Check sheet for the drawn part. Datum: minimum x, y, z corner. Units: mm. A direction names the side the tool comes from. Round coordinates to 2 decimals unless told otherwise and drop trailing zeros. Order: outer loops, then holes, each group sorted by start corner. A loop starts at its lowest first (then second) coordinate and runs counter-clockwise, first axis right, second up. Notation, with made-up numbers: (72, 50) -> (93, 50) arc R21 cw to (93, 65) -> close; hole circle Ø11 at (33.25, 89). An arc over 180 degrees is marked (long way). Answer in a Markdown table with one row per item.
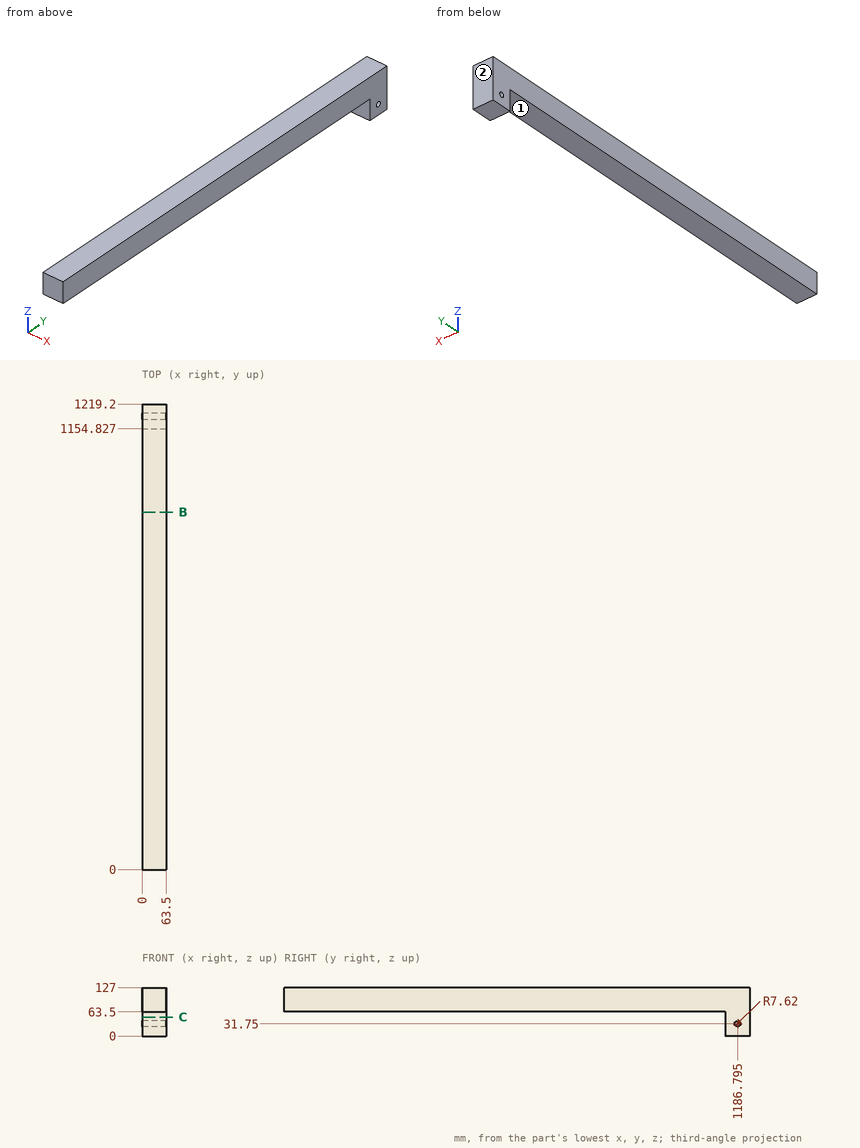
(1) Section check C-C on z = 49.5. Record the boundary of the cut face in (x, y).
Solutions:
| item | result |
|---|---|
| outline | (0, 1154.83) -> (63.5, 1154.83) -> (63.5, 1219.2) -> (0, 1219.2) -> close |
(2) Scan lines: probe 1 along Z at (x, y) = (28, 840); probe 2 along Y at (x, z) = (43.5, 8.5). Record each from-to range of solid material in increasing order. Write a range as from..to.
Solutions:
| item | result |
|---|---|
| probe 1 | 63.5..127 |
| probe 2 | 1154.83..1219.2 |
(3) Depth check by flat-ended pin: pin 1 Ø3 at (x, z) = (14.5, 55.5) entering from -Y; pin 2 Ø2 at (x, y) = (49.5, 322) entering from -Z; pin 3 Ø1.5 at (x, z) = (9, 106) entering from -Y. Enter the tip coordinate at first touch or a pass-through.
Solutions:
| item | result |
|---|---|
| pin 1 | y = 1154.83 |
| pin 2 | z = 63.5 |
| pin 3 | y = 0 |
(4) Section check B-B on y = 936. Record the boundary of the cut face in (x, z), plus the area to 3 significant figures.
Solutions:
| item | result |
|---|---|
| outline | (0, 63.5) -> (63.5, 63.5) -> (63.5, 127) -> (0, 127) -> close |
| area | 4,030 mm^2 |
(5) Tool access check on the marked faces 1 and 2. Record the directions out of +Z, -Z, +X, -X, +Y, -Y that give a thin tool (end or side, any length) a straight path to the whole face; none if there is none.
Solutions:
| item | result |
|---|---|
| face 1 | -Z, +X, -X, -Y |
| face 2 | +Z, -Z, +X, -X, +Y |
